Design review of the part built by this model. Coordinates are the model's own, in mm. A direction names the side the tool comes from. Coordinates: 2 decimals unless noted, no trailing zeros. Write each loop counter-clockwise with the first axis right and the second up, starting at its lowest first coordinate (ties: lowest second). Pieces come first, ordered by that corner, then holes. Notation, with made-up numbers: (69.25, 43) -> (81.25, 43) arc R27 ccw to (81.25, 68) -> close; hole circle Ø11 at (40, 64.25). An arc over 180 degrees is marked (long way). Write item = value, one per line. Start each with the question number.
```python
from build123d import *

# Parameters (mm, degrees)
F0_W     = 75.565
F0_H     = 59.055
F1_DEPTH = 43.18
F2_T     = -2.54
F3_W     = 17.018
F3_H     = 10.541
F4_DEPTH = 3.302
F6_D     = 7.9375
F6_DEPTH = 12.7
F6_TIP   = 2.3846655818
F7_R     = 5.08


# Not quite as in the source:
# - a feature names something its author has since deleted; it is built from what else it names


with BuildPart() as f1:
    # F0 (on Top) → F1 (new body)
    with BuildSketch(Plane.XY):
        Rectangle(F0_W, F0_H)
    extrude(amount=F1_DEPTH)

    # F2
    f2_openings = [f1.faces().sort_by_distance(p)[0] for p in [
        (0, 0, 43.18),
    ]]
    offset(amount=F2_T, openings=f2_openings)

    # F3 (on face) → F4 (cut)
    with BuildSketch(Plane(origin=(0, 29.5275, 0), x_dir=(-1, 0, 0), z_dir=(0, 1, 0))):
        with Locations((19.5056423545, 32.0256687701)):
            Rectangle(F3_W, F3_H)
    extrude(amount=-F4_DEPTH, mode=Mode.SUBTRACT)

    # F6
    with Locations(Plane(origin=(0, 29.5275, 0), x_dir=(-1, 0, 0), z_dir=(0, 1, 0))):
        with Locations((-13.3929288228, 32.0256687701)):
            Hole(F6_D / 2, depth=F6_DEPTH)
            with Locations((0, 0, -(F6_DEPTH + F6_TIP / 2))):  # 118° drill point
                Cone(0, F6_D / 2, F6_TIP, mode=Mode.SUBTRACT)

    # F7
    f7_edges = [f1.edges().sort_by_distance(p)[0] for p in [
        (-37.7825, -29.5275, 21.59),
        (37.7825, -29.5275, 21.59),
        (37.7825, 29.5275, 21.59),
        (-37.7825, 29.5275, 21.59),
    ]]
    fillet(f7_edges, radius=F7_R)


solid = f1.part
```
(1) For faces 1 (the face through (0, 29.528, 21)), 2 (the face through (-10.997, 28, 32)), 3 (the face through (35.242, 0, 23)), list the 3-axis set-ups (+Z, -Z, +X, -X, +Y, -Y) from which the entire face can be reached by the end or side of a thin tool; tool diameter is ignored.
(2) Take a section at B-B, the plane x = 15. State the section outline as (y, z) points.
(3) For line 1 (Y direction, x = -4, z = 9); line 2 (Z direction, x = 13.5, y = 27.5); line 3 (X direction, y = 16, z = 17), list the stretches that pass through material, from the lowest coordinate up.
(4) Mouldability with a two-part tool opening along Z and no side actions: class faces 4 (the face through (-28.015, 28, 32)), 5 (the face through (0, -29.528, 21)), 6 (the face through (0, 29, 43.18)) as pulls with the +Z half, pulls with the -Z half, needs draft (parallel to the pull), parting line crosses it, or undercut.
(5) For pin 1 Ø0.8 at (y, z) = (29, 32.5) entering from +X; pin 2 Ø5 at (x, y) = (3.5, 3.5) entering from +Z; pin 3 Ø0.8 at (y, z) = (28, 30.5) entering from -X, all flat-tipped, find the tip position at first contact; note any pin that passes through.
(6) Take a section at A-A, the plane z = 39. State the section outline as (x, y) points, then the cut area to 3 significant figures.
(7) Take a section at C-C, the plane z = 34. State the section outline as (x, y) points, then the cut area to 3 significant figures.
(8) Take a section at D-D, the plane y = 18.5. State the section outline as (x, z) points.
Report:
q1.face_1 = +Z, -Z, +X, -X, +Y
q1.face_2 = +Y
q1.face_3 = +Z
q2.outline = (-29.53, 0) -> (29.53, 0) -> (29.53, 28.4) -> (26.99, 28.4) -> (26.99, 2.54) -> (-26.99, 2.54) -> (-26.99, 43.18) -> (-29.53, 43.18) -> close; (26.99, 35.65) -> (29.53, 35.65) -> (29.53, 43.18) -> (26.99, 43.18) -> close
q3.line_1 = -29.53 to -26.99, 26.99 to 29.53
q3.line_2 = 0 to 28.06, 35.99 to 43.18
q3.line_3 = -37.78 to -35.24, 35.24 to 37.78
q4.face_4 = undercut
q4.face_5 = needs draft
q4.face_6 = pulls with the +Z half
q5.pin_1 = 35.63
q5.pin_2 = 2.54
q5.pin_3 = -36.69
q6.outline = (-37.78, -24.45) arc R5.08 ccw to (-32.7, -29.53) -> (32.7, -29.53) arc R5.08 ccw to (37.78, -24.45) -> (37.78, 24.45) arc R5.08 ccw to (32.7, 29.53) -> (-32.7, 29.53) arc R5.08 ccw to (-37.78, 24.45) -> close; hole (-35.24, -26.99) -> (35.24, -26.99) -> (35.24, 26.99) -> (-35.24, 26.99) -> close
q6.area = 636 mm2
q7.outline = (-37.78, -24.45) arc R5.08 ccw to (-32.7, -29.53) -> (32.7, -29.53) arc R5.08 ccw to (37.78, -24.45) -> (37.78, 24.45) arc R5.08 ccw to (32.7, 29.53) -> (16.84, 29.53) -> (16.84, 26.99) -> (35.24, 26.99) -> (35.24, -26.99) -> (-35.24, -26.99) -> (-35.24, 26.99) -> (-28.01, 26.99) -> (-28.01, 29.53) -> (-32.7, 29.53) arc R5.08 ccw to (-37.78, 24.45) -> close; (-11, 26.99) -> (9.95, 26.99) -> (9.95, 29.53) -> (-11, 29.53) -> close
q7.area = 575 mm2
q8.outline = (-37.78, 0) -> (37.78, 0) -> (37.78, 43.18) -> (35.24, 43.18) -> (35.24, 2.54) -> (-35.24, 2.54) -> (-35.24, 43.18) -> (-37.78, 43.18) -> close
